Print and shaded views of the part. All mm, measured from the part's lowest x, y and z. A direction names the side the tool comes from. Coordinates: 2 decimals unless noted, no trailing zeros. Loops run counter-clockwise (first coordinate to the right, second up) from the corner with the lowest first, then second, coordinate; pieces in that order, holes last. Notation, with made-up numbers: M -35,52.25 L 19,52.25 A23 cw 19,66.25 Z; hole C 72.25,50.5 d3. An arc over 180 degrees is marked long. Use a Markdown table: item, result. Add a question column.
1) Pin check, flat tip, straight feed: pin 1 Ø1.9 at (x, y) = (9.8, 3) entering from +Z. Stop position of the tip, or through.
2) Tool access for the marked faces 1, 2 and 3: list every direction of +Z, -Z, +X, -X, +Y, -Y with a clear straight run to the whole face (end or side of a thin tool).
3) Pull direction Y, two halves, no side cores. Call the marked faces 4, 5 and 6: released by +Y, released by -Y, zero draft, split by the parting line, or undercut.
4) Band-saw the part on C-C (y = 3). List the corners of the cut face in (x, z) (1 decimal), plus the area to 3 significant figures.
5) Band-saw the part on A-A (z = 5.75). State how many separate pieces and enclosed holes the cut face has.
6) Wall check: probe 1 along Y at (x, z) = (3, 5.25) (1 decimal); probe 2 along Y at (x, z) = (9.8, 4) (1 decimal); probe 3 along Y at (x, z) = (2.5, 8.75). Give the ranges that are in metal, low to high. Write a range as from..to.
7) Band-saw the part on B-B (x = 9.8). List the corners of the cut face in (y, z) (1 decimal).
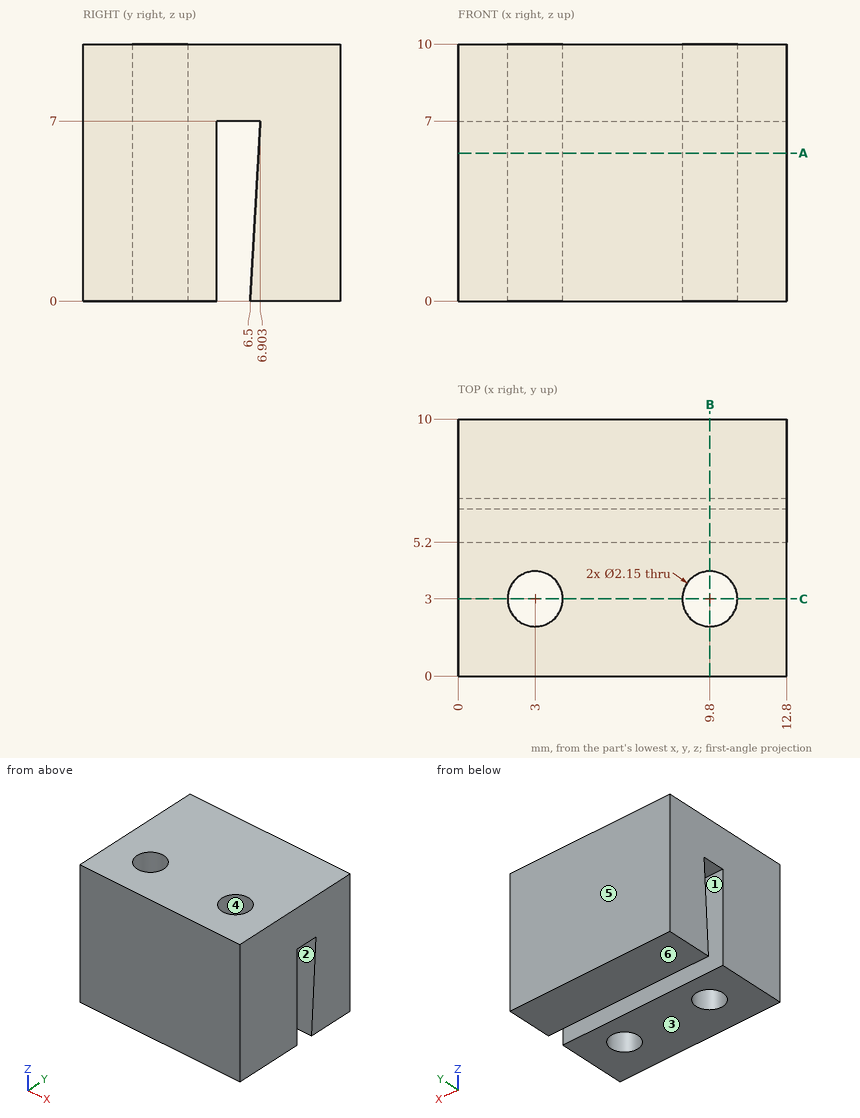
Entries:
| question | item | result |
|---|---|---|
| 1 | pin 1 | through |
| 2 | face 1 | -Z, +X, -X |
| 2 | face 2 | +X, -X |
| 2 | face 3 | -Z, +X, -X, +Y, -Y |
| 3 | face 4 | undercut |
| 3 | face 5 | released by +Y |
| 3 | face 6 | zero draft |
| 4 | outline | M 0,0 L 1.9,0 L 1.9,10 L 0,10 Z; M 4.1,0 L 8.7,0 L 8.7,10 L 4.1,10 Z; M 10.9,0 L 12.8,0 L 12.8,10 L 10.9,10 Z |
| 4 | area | 85.0 mm2 |
| 5 | separate pieces | 2 |
| 5 | enclosed holes | 2 |
| 6 | probe 1 | 0..1.9, 4.1..5.2, 6.8..10 |
| 6 | probe 2 | 0..1.9, 4.1..5.2, 6.7..10 |
| 6 | probe 3 | 0..2.05, 3.95..10 |
| 7 | outline | M 0,0 L 1.9,0 L 1.9,10 L 0,10 Z; M 4.1,0 L 5.2,0 L 5.2,7 L 6.9,7 L 6.5,0 L 10,0 L 10,10 L 4.1,10 Z |
